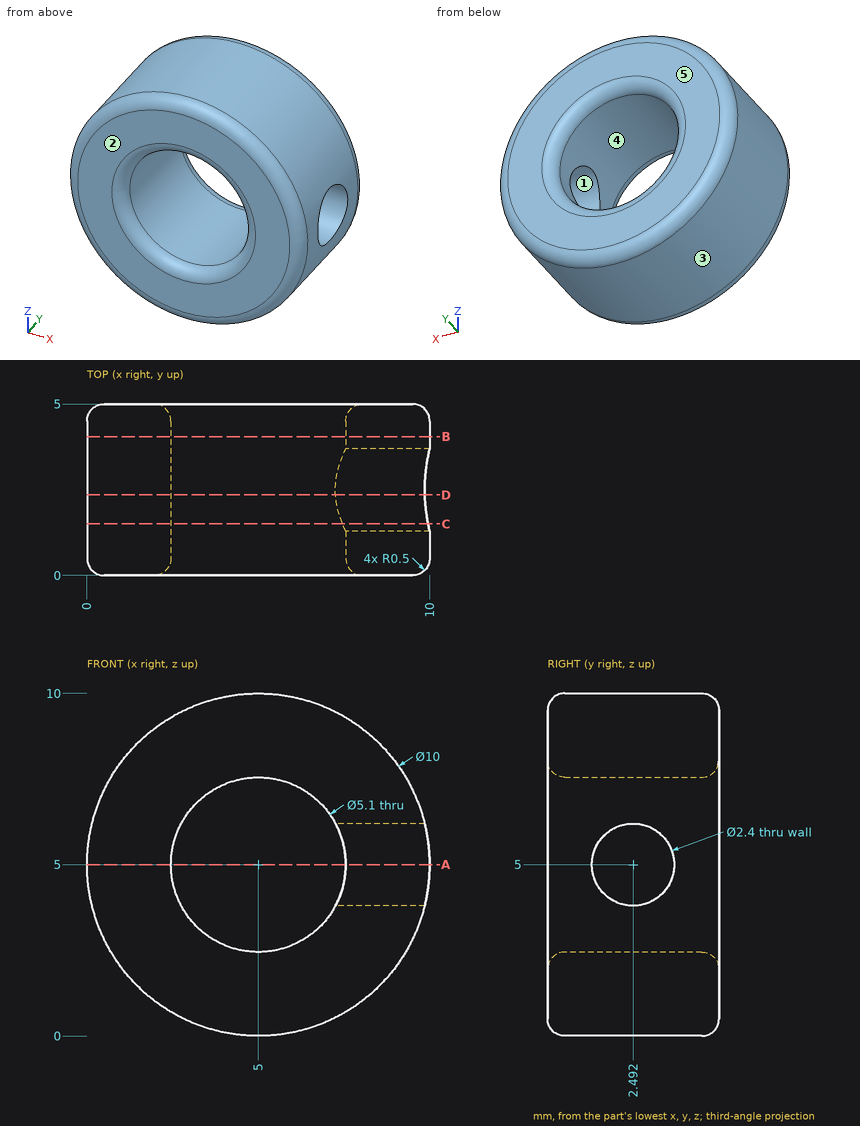
Drawing for the job (mm, zero at the part's lowest x, y, z). A direction names the side the tool comes from. Give positions to 0.01 mm unless a question says otherwise; leave off trailing zeros. Order: outer loops, then holes, each group sorted by start corner. A loop starts at its lowest first (then second) coordinate and runs counter-clockwise, first axis right, second up. Notation, with made-up numbers: M 38.25,-8.5 L 72.25,-8.5 A26 ccw 72.25,5.5 Z; hole C 83.25,-27.75 d9. An arc over 180 degrees is marked long. Use a Markdown table: item, result. Add a question column.
(1) Drop flat-ended pins along their axis: P1, Ø1, axis at x = 1.5, y = 1, coming from the -Z side; P2, Ø2, axis at x = 1.5, y = 4.5, coming from the +Z side. Give the stop position or say it passes through.
(2) Probe line 1 along X through (y, z) = (1.2, 5); line 2 along X through (y, z) = (3.2, 5); line 3 along Y through (x, z) = (9.4, 5). List the from-to ranges inside material, lowest first. Write a range as [from, to].
(3) Saw through at A-A, the plane z = 5. Give the number of separate pieces and of enclosed holes in the cut face, and give its area (3 significant figures).
(4) Mould opens along Z. For the marked faces 3, 4 and 5 say: +Z half, -Z half, draft (parallel to the pull), parting line (faces both ways), or undercut.
(5) Saw through at D-D, the plane y = 2.35. Give the cut face in (x, z).
(6) 3-axis set-ups, long thin cutter, end or side, ignore diameter. For the marked faces 1 and 2: which of +Z, -Z, +X, -X, +Y, -Y reach the whole face in a straight line?
(7) Saw through at C-C, the plane y = 1.5. Give the cut face in (x, z).
(8) Saw through at B-B, the plane y = 4.05. Give the cut face in (x, z), and give its area (3 significant figures).
Answer key:
| question | item | result |
|---|---|---|
| 1 | P1 | z = 1 |
| 1 | P2 | z = 9.33 |
| 2 | line 1 | [0, 2.45], [7.55, 10] |
| 2 | line 2 | [0, 2.45] |
| 2 | line 3 | [0, 1.29], [3.69, 5] |
| 3 | separate pieces | 3 |
| 3 | enclosed holes | 0 |
| 3 | area | 18.2 mm^2 |
| 4 | face 3 | parting line |
| 4 | face 4 | undercut |
| 4 | face 5 | draft |
| 5 | outline | M 7.25,3.81 A2.55 cw long 7.25,6.19 L 9.86,6.19 A5 ccw long 9.86,3.81 Z |
| 6 | face 1 | +X |
| 6 | face 2 | +Z, -Z, +X, -X, -Y |
| 7 | outline | M 7.46,4.32 A2.55 cw long 7.46,5.68 L 9.95,5.68 A5 ccw long 9.95,4.32 Z |
| 8 | outline | C 5,5 d10; hole C 5,5 d5.1 |
| 8 | area | 58.1 mm^2 |
